The listing builds one solid part. Answer for the finished solid, in the listing's coordinates (mm). Face numbers are marked on the shaded views. A direction names the side the tool comes from. Coordinates: 2 decimals unless noted, no trailing zeros. Order: outer loops, then holes, each group sorted by start corner. A loop starts at its lowest first (then second) coordinate and runs counter-clockwise, first axis right, second up.
from build123d import *

# Parameters (mm, degrees)
SKETCH_W     = 45
SKETCH_H     = 25
PAD_DEPTH    = 2.5
SKETCH001_R  = 1.6
POCKET_DEPTH = 5
SKETCH002_W  = 10
SKETCH002_H  = 1
PAD001_DEPTH = 5


with BuildPart() as part:
    # Sketch → Pad (new body)
    with BuildSketch(Plane.XY):
        Rectangle(SKETCH_W, SKETCH_H)
    extrude(amount=PAD_DEPTH)

    # Sketch001 → Pocket (cut)
    with BuildSketch(Plane.XY.offset(2.5)):
        with Locations((18, -8)):
            Circle(SKETCH001_R)
        with BuildLine():
            ThreePointArc((-17.5, 5.3), (-19.3, 3.5), (-17.5, 1.7))
            Line((-17.5, 1.7), (17.5, 1.7))
            ThreePointArc((17.5, 1.7), (19.3, 3.5), (17.5, 5.3))
            Line((-17.5, 5.3), (17.5, 5.3))
        make_face()
    extrude(amount=-POCKET_DEPTH, mode=Mode.SUBTRACT)

    # Sketch002 → Pad001 (new body)
    with BuildSketch(Plane(origin=(0, 0, 0), x_dir=(1, 0, 0), z_dir=(0, 0, -1))):
        with Locations((17.5, 3)):
            Rectangle(SKETCH002_W, SKETCH002_H)
    extrude(amount=PAD001_DEPTH)


solid = part.part
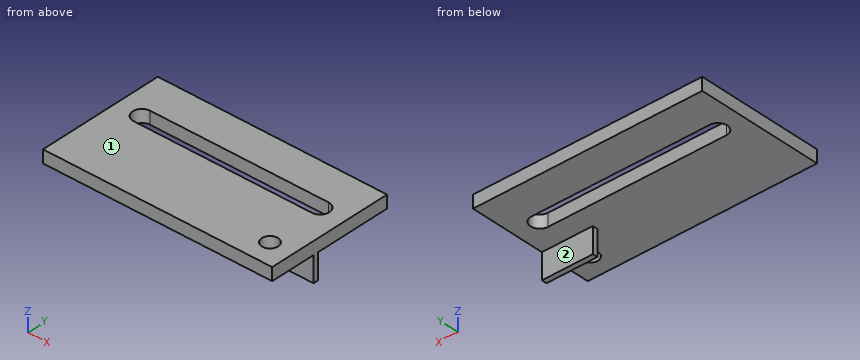
1) Each of these flat-tipped pins is pushed along its axis until it touches: P1, Ø2.5, axis at x = 18, z = -3, coming from the -Y side; P2, Ø0.8, axis at y = -3, z = -1.5, coming from the -X side; P3, Ø4, axis at x = -12, y = -1, coming from the -Z side. Where does it stop, or does it pass through?
2) Section B-B (y = 3.5) is taken. Give the vertices of the cut face in (x, z).
3) Consider L1, parallel to Y at x = 18, z = 1; L2, parallel to Y at x = -4, z = 0.5; L3, parallel to Z at x = -13, y = 11.25. Determine where each line is inside the solid, lowest interval first.
4) Section D-D (x = 20.5) is taken. Give the vertices of the cut face in (y, z).
5) Section A-A (x = 15) is taken. Give the vertices of the cut face in (y, z), then the cut area to 3 significant figures.
6) Section C-C (x = -3) is taken. Give the vertices of the cut face in (y, z).
7) A tool of negligible diameter and unlimited length cuts with its end or side. For the marked faces 1 and 2, from which of +Z, -Z, +X, -X, +Y, -Y can it reach the whole face along a straight path? Write none if from no direction.
Filled sheet:
1. P1: stops at y = -3.5
1. P2: stops at x = 12.5
1. P3: stops at z = 0
2. outline: (-22.5, 0) - (-19.3, 0) - (-19.3, 2.5) - (-22.5, 2.5) - close; (19.3, 0) - (22.5, 0) - (22.5, 2.5) - (19.3, 2.5) - close
3. L1: y = -12.5 to -9.6, -6.4 to 1.77, 5.23 to 12.5
3. L2: y = -12.5 to 1.7, 5.3 to 12.5
3. L3: z = 0 to 2.5
4. outline: (-12.5, 0) - (-3.5, 0) - (-3.5, -5) - (-2.5, -5) - (-2.5, 0) - (12.5, 0) - (12.5, 2.5) - (-12.5, 2.5) - close
5. outline: (-12.5, 0) - (-3.5, 0) - (-3.5, -5) - (-2.5, -5) - (-2.5, 0) - (1.7, 0) - (1.7, 2.5) - (-12.5, 2.5) - close; (5.3, 0) - (12.5, 0) - (12.5, 2.5) - (5.3, 2.5) - close
5. area: 58.5 mm2
6. outline: (-12.5, 0) - (1.7, 0) - (1.7, 2.5) - (-12.5, 2.5) - close; (5.3, 0) - (12.5, 0) - (12.5, 2.5) - (5.3, 2.5) - close
7. face 1: +Z, +X, -X, +Y, -Y
7. face 2: -Z, +X, -X, +Y
